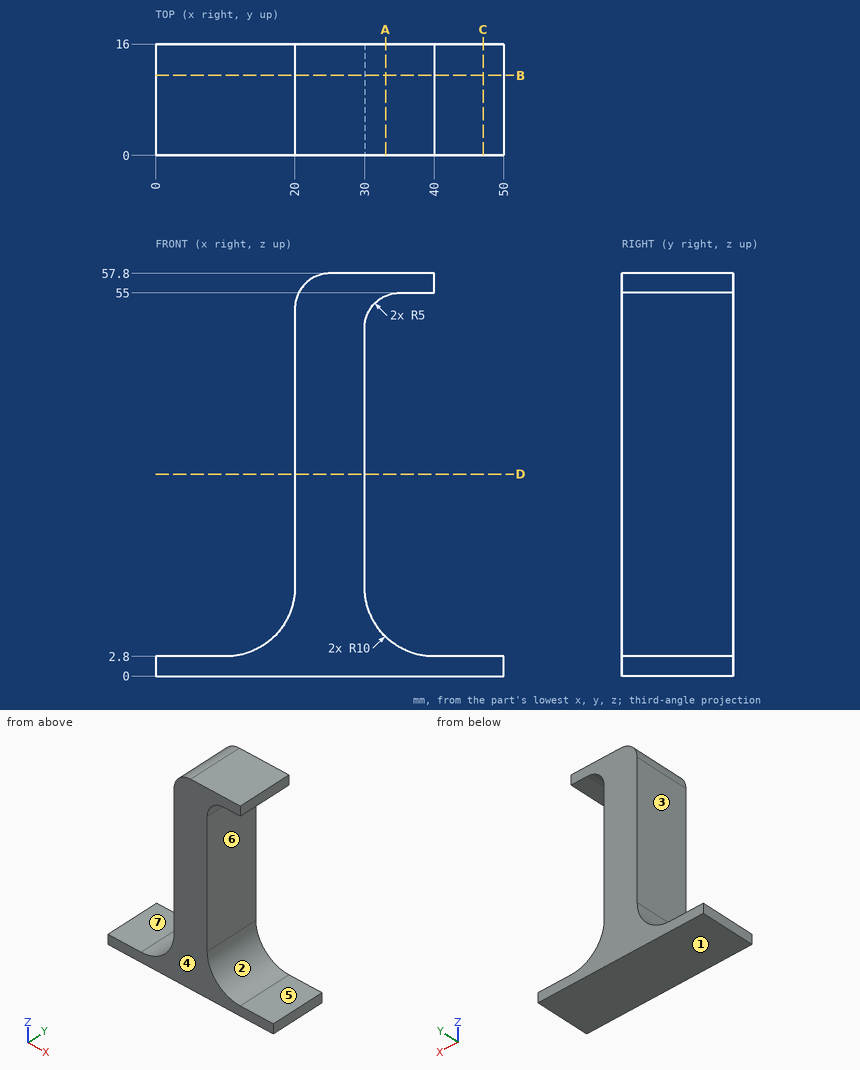
The figure shows three views and two pictorial views of one solid part (mm, origin at its lowest corner). Answer the questions. A direction names the side the tool comes from. Give positions to 0.01 mm unless a question says otherwise; leave off trailing zeros. Loops run counter-clockwise (first coordinate to the right, second up) from the corner with the lowest first, then second, coordinate; pieces in that order, holes last. Notation, with made-up numbers: (12.25, 79.25) -> (37.25, 79.25) arc R23 cw to (37.25, 87.25) -> close; hole circle Ø1 at (82.25, 2). An arc over 180 degrees is marked (long way). Use CSV: the item, a comma, the result in double quotes.
1. The part is cut by section A-A (x = 33). Write down the section's boundary in (y, z).
Found:
outline,"(0, 0) -> (16, 0) -> (16, 5.66) -> (0, 5.66) -> close; (0, 54.58) -> (16, 54.58) -> (16, 57.8) -> (0, 57.8) -> close"
2. Straight lines are drawn through the part: line 1 (X direction, y = 1.25, z = 48.5); line 2 (Z direction, x = 4.5, y = 1.5); line 3 (Z direction, x = 36.5, y = 7.25). For each, find the intervals that lie inside material, in ascending order.
Found:
line 1,"20 to 30"
line 2,"0 to 2.8"
line 3,"0 to 3.43, 55 to 57.8"
3. The part is cut by section B-B (y = 11.5). Write down the section's boundary in (x, z).
Found:
outline,"(0, 0) -> (50, 0) -> (50, 2.8) -> (40, 2.8) arc R10 cw to (30, 12.8) -> (30, 50) arc R5 cw to (35, 55) -> (40, 55) -> (40, 57.8) -> (25, 57.8) arc R5 ccw to (20, 52.8) -> (20, 12.8) arc R10 cw to (10, 2.8) -> (0, 2.8) -> close"
4. The part is cut by section C-C (x = 47). Write down the section's boundary in (y, z).
Found:
outline,"(0, 0) -> (16, 0) -> (16, 2.8) -> (0, 2.8) -> close"
5. Flat-ended cylindrical pins translate along their axes: pin 1 Ø5 at (x, y) = (45.5, 7.5) entering from +Z; pin 2 Ø5 at (y, z) = (7, 15) entering from +X; pin 3 Ø1.5 at (y, z) = (2.5, 7.5) entering from +X. Find the tip coordinate at first contact, or state that the pin passes through.
Found:
pin 1,"z = 2.8"
pin 2,"x = 30"
pin 3,"x = 32.04"
6. A tool of negligible diameter and unlimited length cuts with its end or side. For the marked faces 4, 5, 6 and 7, from which of +Z, -Z, +X, -X, +Y, -Y can it reach the whole face along a straight path? Write none if from no direction.
Found:
face 4,"+Z, -Z, +X, -X, -Y"
face 5,"+Z, +X, +Y, -Y"
face 6,"+X, +Y, -Y"
face 7,"+Z, -X, +Y, -Y"
7. The mould has two halves that part along Z. Classify the marked faces 1, 2 and 3: +Z half, -Z half, draft (parallel to the pull), parting line (faces both ways), or undercut.
Found:
face 1,"-Z half"
face 2,"undercut"
face 3,"draft"
8. The part is cut by section D-D (z = 29). Write down the section's boundary in (x, y), then the cut area to 3 significant figures.
Found:
outline,"(20, 0) -> (30, 0) -> (30, 16) -> (20, 16) -> close"
area,"160 mm^2"
